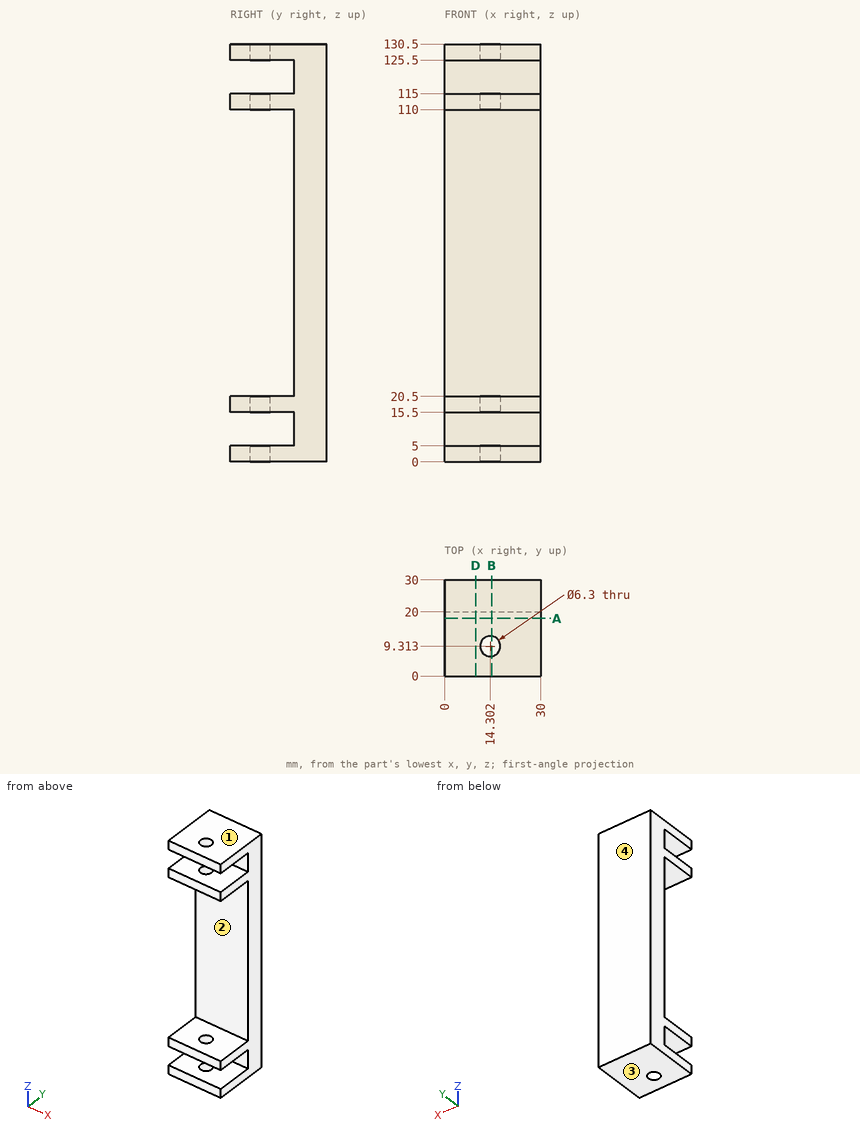
Can you work these out from the drawing? Everything is in mm from the part's minimum corner. Round coordinates to 2 decimals unless told otherwise and drop trailing zeros. Write each loop counter-clockwise with the first axis right and the second up, starting at its lowest first coordinate (ties: lowest second). Pieces come first, ordered by that corner, then holes.
1. Suppose I cut it at B-B (x = 14.75). State how many separate pieces and enclosed holes the cut face has, and give its area (3 significant figures).
2. Suppose I cut it at D-D (x = 9.75). List the corners of the cut face in (y, z) for me.
3. If we mould it in two halves opening along Z, with no side actions, what happens to the marked faces 1, 2, 3 and 4? For each: released by +Z, released by -Z, zero draft, split by the parting line, or undercut.
4. Suppose I cut it at A-A (y = 18). List the corners of the cut face in (x, z) for me.
5. I need wall thicknesses on L1, parallel to Z at x = 23.5, y = 10; L2, parallel to Y at x = 4.5, z = 24; L3, parallel to X at y = 12, z = 112 (1 decimal). Which ranges of each line are inside material? Lowest first, please.
6. Will these pins go through, and if not, where does the flat tip stop? pin 1 Ø1 at (x, z) = (15, 106) entering from -Y; pin 2 Ø4 at (x, y) = (14.3, 9.31) entering from -Z.
Answer sheet:
1. separate pieces: 5
1. enclosed holes: 0
1. area: 1,580 mm2
2. outline: (0, 0) - (30, 0) - (30, 130.5) - (0, 130.5) - (0, 125.5) - (20, 125.5) - (20, 115) - (0, 115) - (0, 110) - (20, 110) - (20, 20.5) - (0, 20.5) - (0, 15.5) - (20, 15.5) - (20, 5) - (0, 5) - close
3. face 1: released by +Z
3. face 2: undercut
3. face 3: released by -Z
3. face 4: zero draft
4. outline: (0, 0) - (30, 0) - (30, 5) - (0, 5) - close; (0, 15.5) - (30, 15.5) - (30, 20.5) - (0, 20.5) - close; (0, 110) - (30, 110) - (30, 115) - (0, 115) - close; (0, 125.5) - (30, 125.5) - (30, 130.5) - (0, 130.5) - close
5. L1: z = 0 to 5, 15.5 to 20.5, 110 to 115, 125.5 to 130.5
5. L2: y = 20 to 30
5. L3: x = 0 to 12.7, 15.9 to 30
6. pin 1: stops at y = 20
6. pin 2: passes through
